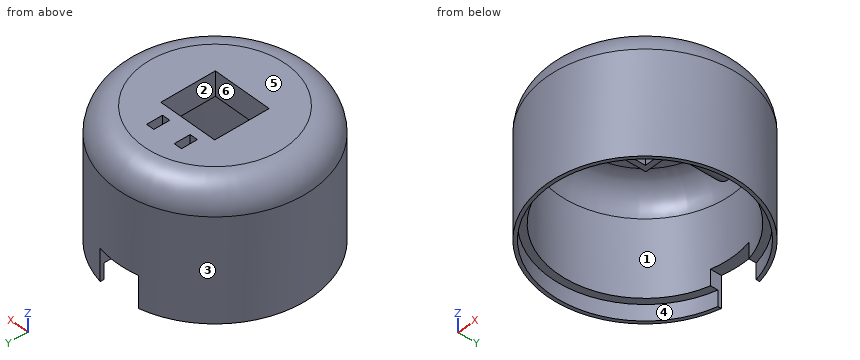
from build123d import *

# Parameters (mm, degrees)
F0_R      = 18.5
F1_DEPTH  = 24.4
F2_T      = -2
F3_R      = 5
F4_R      = 5
F5_W      = 11.2
F5_H      = 10.3
F6_DEPTH  = 25
F7_W      = 8
F7_H      = 32.8909642994
F8_DEPTH  = 6
F9_R      = 17.85
F10_DEPTH = 3
F5_W_2    = 13.2
F5_H_2    = 12.3
F11_DEPTH = 4.6
F13_DEPTH = 10
F14_W     = 1.5
F14_H     = 3
F15_DEPTH = 25


with BuildPart() as f1:
    # F0 (on Top) → F1 (new body)
    with BuildSketch(Plane.XY):
        Circle(F0_R)
    extrude(amount=F1_DEPTH)

    # F2
    f2_openings = [f1.faces().sort_by_distance(p)[0] for p in [
        (0, 0, 0),
    ]]
    offset(amount=F2_T, openings=f2_openings)

    # F3
    f3_edges = [f1.edges().sort_by_distance(p)[0] for p in [
        (-16.5, 0, 22.4),
    ]]
    fillet(f3_edges, radius=F3_R)

    # F4
    f4_edges = [f1.edges().sort_by_distance(p)[0] for p in [
        (-18.5, 0, 24.4),
    ]]
    fillet(f4_edges, radius=F4_R)

    # F5 (on face) → F6 (cut)
    with BuildSketch(Plane.XY.offset(24.4)):
        Rectangle(F5_W, F5_H)
    extrude(amount=-F6_DEPTH, mode=Mode.SUBTRACT)

    # F7 (on face) → F8 (cut)
    with BuildSketch(Plane(origin=(0, 0, 0), x_dir=(1, 0, 0), z_dir=(0, 0, -1))):
        with Locations((0, -3.944914788)):
            Rectangle(F7_W, F7_H)
    extrude(amount=-F8_DEPTH, mode=Mode.SUBTRACT)

    # F9 (on face) + F7 (on face) → F10 (cut)
    with BuildSketch(Plane(origin=(0, 0, 0), x_dir=(1, 0, 0), z_dir=(0, 0, -1))):
        Circle(F9_R)
    with BuildSketch(Plane(origin=(0, 0, 0), x_dir=(1, 0, 0), z_dir=(0, 0, -1))):
        with Locations((0, -3.944914788)):
            Rectangle(F7_W, F7_H)
    extrude(amount=-F10_DEPTH, mode=Mode.SUBTRACT)

    # F5 (on face) → F11 (join)
    with BuildSketch(Plane.XY.offset(24.4)):
        Rectangle(F5_W_2, F5_H_2)
        Rectangle(F5_W, F5_H, mode=Mode.SUBTRACT)
    extrude(amount=-F11_DEPTH)

    # F12 (on face) → F13 (join)
    with BuildSketch(Plane(origin=(0, 6.15, 0), x_dir=(-1, 0, 0), z_dir=(0, 1, 0))):
        with BuildLine():
            Line((2.4086248595, 22.4), (-1.8398975953, 22.4))
            ThreePointArc((-1.8398975953, 22.4), (0.2843636321, 19.8238066567), (2.4086248595, 22.4))
        make_face()
    extrude(amount=F13_DEPTH)

    # F14 (on face) → F15 (cut)
    with BuildSketch(Plane(origin=(0, 0, 22.4), x_dir=(1, 0, 0), z_dir=(0, 0, -1))):
        with Locations((-3.1586248595, -8.3878219724)):
            Rectangle(F14_W, F14_H)
        with Locations((2.5898975953, -8.3878219724)):
            Rectangle(F14_W, F14_H)
    extrude(amount=-F15_DEPTH, mode=Mode.SUBTRACT)


solid = f1.part
Can you work these out from the model? Positions are in its coordinate system, mm. Face numbers are marked on the shaded views. A direction names the side the tool comes from. Coordinates: 2 decimals unless noted, no trailing zeros. Loops run counter-clockwise (first coordinate to the right, second up) from the corner with the lowest first, then second, coordinate; pieces in that order, holes last. Notation, with made-up numbers: (36.5, 41.25) - (87.5, 41.25) arc R25 ccw to (87.5, 79.25) - close; hole circle Ø1 at (-1.5, 79.25). An arc over 180 degrees is marked (long way). Put each result on its own line as item: value. Start each with the question number.
Item 1: Suppose I cut it at B-B (x = 0). Please give me the cut outline in (y, z), and give its area (3 significant figures).
Item 2: If we mould it in two halves opening along Y, with no side actions, what happens to the marked faces 3, 4, 5 and 6? For each: +Y half, -Y half, draft (parallel to the pull), parting line (faces both ways), or undercut.
Item 3: For pin 1 (1.6 mm diameter, centred on y = 9, z = 24, fed in from +X); pin 2 (7 mm diameter, centred on x = 5.5, y = 0, fed in from -Z); pin 3 (1.3 mm diameter, centred on y = 0.5, z = 20.5, fed in from -X); pin 4 (8 mm diameter, centred on y = -0.5, z = 3, fed in from +X), each with a flat end and sliding along its axis, tell me the tip position at first contact or that it passes through.
Item 4: Suppose I cut it at C-C (z = 12.5). Please give me the cut outline in (x, y).
Item 5: Which directions (+Z, -Z, +X, -X, +Y, -Y) give clear straight access to the entire face, cutting with the end or side of a thin tool? Please do the marked faces 1 and 2.
Item 6: Suppose I cut it at D-D (y = 7.5). State how many separate pieces and enclosed holes the cut face has, and give its area (3 significant figures).
Item 7: Suppose I cut it at A-A (y = 0). Please give me the cut outline in (x, z), and give its area (3 significant figures).
Item 8: If I drill on line 1 along X through (y, z) = (0, 0.7); line 2 along Y through (x, z) = (0, 11.25); line 3 along Y through (x, z) = (5, 20.75), over which ranges is the centre line in solid material (lowest first)?
Here are the results:
1. outline: (-18.5, 0) - (-17.85, 0) - (-17.85, 3) - (-16.5, 3) - (-16.5, 17.4) arc R5 cw to (-11.5, 22.4) - (-6.15, 22.4) - (-6.15, 19.8) - (-5.15, 19.8) - (-5.15, 24.4) - (-13.5, 24.4) arc R5 ccw to (-18.5, 19.4) - close; (5.15, 19.8) - (6.15, 19.8) - (6.15, 19.84) - (15.86, 19.84) arc R5 cw to (16.5, 17.4) - (16.5, 6) - (18.5, 6) - (18.5, 19.4) arc R5 ccw to (13.5, 24.4) - (5.15, 24.4) - close
1. area: 154 mm²
2. face 3: parting line
2. face 4: undercut
2. face 5: draft
2. face 6: undercut
3. pin 1: x = 14.23
3. pin 2: z = 19.8
3. pin 3: x = -18.47
3. pin 4: x = 18.5
4. outline: circle Ø37 at (0, 0); hole circle Ø33 at (0, 0)
5. face 1: -Z
5. face 2: +Z, -Z
6. separate pieces: 3
6. enclosed holes: 0
6. area: 161 mm²
7. outline: (-18.5, 0) - (-17.85, 0) - (-17.85, 3) - (-16.5, 3) - (-16.5, 17.4) arc R5 cw to (-11.5, 22.4) - (-6.6, 22.4) - (-6.6, 19.8) - (-5.6, 19.8) - (-5.6, 24.4) - (-13.5, 24.4) arc R5 ccw to (-18.5, 19.4) - close; (5.6, 19.8) - (6.6, 19.8) - (6.6, 22.4) - (11.5, 22.4) arc R5 cw to (16.5, 17.4) - (16.5, 3) - (17.85, 3) - (17.85, 0) - (18.5, 0) - (18.5, 19.4) arc R5 ccw to (13.5, 24.4) - (5.6, 24.4) - close
7. area: 138 mm²
8. line 1: -18.5 to -17.85, 17.85 to 18.5
8. line 2: -18.5 to -16.5, 16.5 to 18.5
8. line 3: -17.62 to -14.37, -6.15 to -5.15, 5.15 to 6.15, 14.37 to 17.62
